Here's how the part is built. I have some questions about the finished solid (model axes, mm). Face numbers are marked on the shaded views. A direction names the side the tool comes from. Coordinates: 2 decimals unless noted, no trailing zeros. Write each loop counter-clockwise with the first axis right and the second up, starting at its lowest first coordinate (ties: lowest second). Pieces come first, ordered by that corner, then holes. Notation, with made-up numbers: (-18.75, 56) -> (5.25, 56) arc R11 cw to (5.25, 65) -> close; hole circle Ø8 at (70, -15.75). An arc over 180 degrees is marked (long way). Use CSV: the item, a comma, the result in double quotes. Start each with the question number.
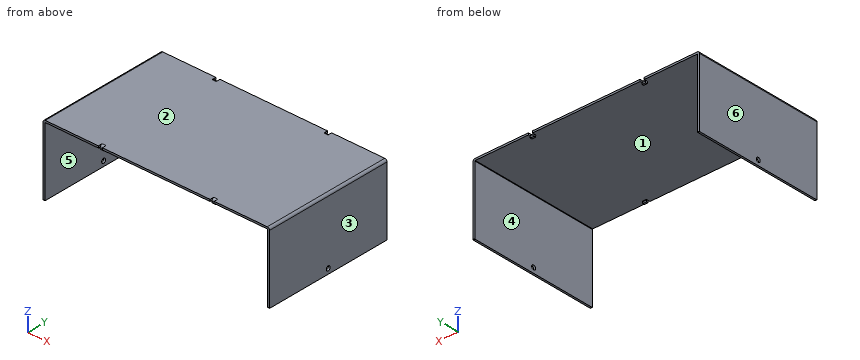
```python
from build123d import *

# Parameters (mm, degrees)
SKETCH1_W                      = 152.4
SKETCH1_H                      = 88.9
BASE_FLANGE1_DEPTH             = 1.29032
EDGE_FLANGE1_STRIP_W           = 5.85978
EDGE_FLANGE1_STRIP_H           = 1.29032
EDGE_FLANGE1_STRIP_CUT_DEPTH   = 88.9
EDGE_FLANGE1_STRIP_2_W         = 5.85978
EDGE_FLANGE1_STRIP_2_H         = 1.29032
EDGE_FLANGE1_STRIP_CUT_2_DEPTH = 88.9
EDGE_FLANGE1_DEPTH             = 88.9
EDGE_FLANGE1_BEND_DEPTH        = 88.9
M3X0_5_TAPPED_HOLE1_REACH      = 170.648
M3X0_5_TAPPED_HOLE1_BORE_R     = 1.5
BREAK_CORNER1_START            = -77.68082
BREAK_CORNER1_DEPTH            = 155.36164
CUT_THICKEN1_START             = 41.91
CUT_THICKEN1_OUTLINE_W         = 0.127
CUT_THICKEN1_OUTLINE_H         = 1.29032
CUT_THICKEN1_DEPTH             = 2.54
CUT_THICKEN2_START             = 41.91
CUT_THICKEN2_OUTLINE_W         = 0.127
CUT_THICKEN2_OUTLINE_H         = 1.29032
CUT_THICKEN2_DEPTH             = 2.54
MIRROR7_START                  = 41.91
MIRROR7_COPY_1_SKETCH_W        = 0.127
MIRROR7_COPY_1_SKETCH_H        = 1.29032
MIRROR7_COPY_1_DEPTH           = 2.54
MIRROR7_COPY_2_SKETCH_W        = 0.127
MIRROR7_COPY_2_SKETCH_H        = 1.29032
MIRROR7_COPY_2_DEPTH           = 2.54
MOVE_FACE1_BY                  = 1.27
MOVE_FACE1_2_BY                = 1.27
MOVE_FACE1_3_BY                = 1.27
MOVE_FACE1_4_BY                = 1.27
EDGE_FLANGE2_STRIP_W           = 5.66928
EDGE_FLANGE2_STRIP_H           = 1.29032
EDGE_FLANGE2_STRIP_CUT_DEPTH   = 2.54
EDGE_FLANGE2_STRIP_2_W         = 5.66928
EDGE_FLANGE2_STRIP_2_H         = 1.29032
EDGE_FLANGE2_STRIP_CUT_2_DEPTH = 2.54
EDGE_FLANGE2_STRIP_3_W         = 5.66928
EDGE_FLANGE2_STRIP_3_H         = 1.29032
EDGE_FLANGE2_STRIP_CUT_3_DEPTH = 2.54
EDGE_FLANGE2_STRIP_4_W         = 5.66928
EDGE_FLANGE2_STRIP_4_H         = 1.29032
EDGE_FLANGE2_STRIP_CUT_4_DEPTH = 2.54
EDGE_FLANGE2_DEPTH             = 2.54
EDGE_FLANGE2_BEND_DEPTH        = 2.54
EDGE_FLANGE2_BEND_2_DEPTH      = 2.54
EDGE_FLANGE2_BEND_3_DEPTH      = 2.54


# Read off the part's stored shape, not the designer's step: Break-Corner1, Cut-Thicken1, Cut-Thicken2
# Sheet-metal steps are written as plain solids
with BuildPart() as part:
    # Sketch1 → Base-Flange1 (new body)
    with BuildSketch(Plane.XY):
        Rectangle(SKETCH1_W, SKETCH1_H)
    extrude(amount=-BASE_FLANGE1_DEPTH)

    # Edge-Flange1 strip (across the edge) → Edge-Flange1 strip cut (cut)
    with BuildSketch(Plane(origin=(-76.3905, -44.45, -1.29032), x_dir=(1, 0, 0), z_dir=(0, 1, 0))):
        with Locations((-2.67589, -0.64516)):
            Rectangle(EDGE_FLANGE1_STRIP_W, EDGE_FLANGE1_STRIP_H)
    extrude(amount=EDGE_FLANGE1_STRIP_CUT_DEPTH, mode=Mode.SUBTRACT)

    # Edge-Flange1 strip 2 (across the edge) → Edge-Flange1 strip cut 2 (cut)
    with BuildSketch(Plane(origin=(76.3905, 44.45, -1.29032), x_dir=(-1, 0, 0), z_dir=(0, -1, 0))):
        with Locations((-2.67589, -0.64516)):
            Rectangle(EDGE_FLANGE1_STRIP_2_W, EDGE_FLANGE1_STRIP_2_H)
    extrude(amount=EDGE_FLANGE1_STRIP_CUT_2_DEPTH, mode=Mode.SUBTRACT)

    # Edge-Flange1 section (across the edge) → Edge-Flange1 (add)
    with BuildSketch(Plane(origin=(-76.3905, -44.45, -1.29032), x_dir=(1, 0, 0), z_dir=(0, 1, 0))):
        with BuildLine():
            Line((-1.29032, 0.254), (-1.29032, 46.96968))
            Line((-1.29032, 46.96968), (0, 46.96968))
            Line((0, 46.96968), (0, 0.254))
            ThreePointArc((0, 0.254), (0.074394878, 0.074394878), (0.254, 0))
            Line((0.254, 0), (0.254, -1.29032))
            ThreePointArc((0.254, -1.29032), (-0.837999144, -0.837999144), (-1.29032, 0.254))
        make_face()
    extrude(amount=EDGE_FLANGE1_DEPTH)

    # Edge-Flange1 section 2 (across the edge) → Edge-Flange1 bend (add)
    with BuildSketch(Plane(origin=(76.3905, 44.45, -1.29032), x_dir=(-1, 0, 0), z_dir=(0, -1, 0))):
        with BuildLine():
            Line((-1.29032, 0.254), (-1.29032, 46.96968))
            Line((-1.29032, 46.96968), (0, 46.96968))
            Line((0, 46.96968), (0, 0.254))
            ThreePointArc((0, 0.254), (0.074394878, 0.074394878), (0.254, 0))
            Line((0.254, 0), (0.254, -1.29032))
            ThreePointArc((0.254, -1.29032), (-0.837999144, -0.837999144), (-1.29032, 0.254))
        make_face()
    extrude(amount=EDGE_FLANGE1_BEND_DEPTH)

    # M3x0.5 Tapped Hole1 bore → M3x0.5 Tapped Hole1 (cut, up to next)
    with BuildSketch(Plane.ZY.offset(77.68082), mode=Mode.PRIVATE) as m3x0_5_tapped_hole1_sk1:
        with Locations((-44.7675, 0)):
            Circle(M3X0_5_TAPPED_HOLE1_BORE_R)
    m3x0_5_tapped_hole1_tool1 = extrude(m3x0_5_tapped_hole1_sk1.sketch, amount=-M3X0_5_TAPPED_HOLE1_REACH, mode=Mode.PRIVATE) & part.part
    m3x0_5_tapped_hole1 = m3x0_5_tapped_hole1_tool1.solids().sort_by_distance((-77.68082, 0, -44.7675))[0]
    add(m3x0_5_tapped_hole1, mode=Mode.SUBTRACT)

    # Mirror1: M3x0.5 Tapped Hole1 across plane
    add(m3x0_5_tapped_hole1.mirror(Plane(origin=(0, 0, 0), x_dir=(0, 0, 1), z_dir=(1, 0, 0))), mode=Mode.SUBTRACT)

    # Break-Corner1 outline → Break-Corner1 (cut)
    with BuildSketch(Plane.YZ.offset(BREAK_CORNER1_START)):
        with BuildLine():
            Line((44.45, -48.26), (44.45, -48.006))
            ThreePointArc((44.45, -48.006), (44.375605122, -48.185605122), (44.196, -48.26))
            Line((44.196, -48.26), (44.45, -48.26))
        make_face()
        with BuildLine():
            Line((-44.45, -48.26), (-44.196, -48.26))
            ThreePointArc((-44.196, -48.26), (-44.375605122, -48.185605122), (-44.45, -48.006))
            Line((-44.45, -48.006), (-44.45, -48.26))
        make_face()
    extrude(amount=BREAK_CORNER1_DEPTH, mode=Mode.SUBTRACT)

    # Cut-Thicken1 outline → Cut-Thicken1 (cut)
    with BuildSketch(Plane(origin=(0, 0, 0), x_dir=(1, 0, 0), z_dir=(0, 1, 0)).offset(CUT_THICKEN1_START)):
        with Locations((36.97732, 0.64516)):
            Rectangle(CUT_THICKEN1_OUTLINE_W, CUT_THICKEN1_OUTLINE_H)
    cut_thicken1 = extrude(amount=CUT_THICKEN1_DEPTH, mode=Mode.SUBTRACT)

    # Cut-Thicken2 outline → Cut-Thicken2 (cut)
    with BuildSketch(Plane(origin=(0, 0, 0), x_dir=(1, 0, 0), z_dir=(0, 1, 0)).offset(CUT_THICKEN2_START)):
        with Locations((39.64432, 0.64516)):
            Rectangle(CUT_THICKEN2_OUTLINE_W, CUT_THICKEN2_OUTLINE_H)
    cut_thicken2 = extrude(amount=CUT_THICKEN2_DEPTH, mode=Mode.SUBTRACT)

    # Mirror6: Cut-Thicken1, Cut-Thicken2 across plane
    add(cut_thicken1.mirror(Plane(origin=(0, 0, 0), x_dir=(0, 0, 1), z_dir=(1, 0, 0))), mode=Mode.SUBTRACT)
    add(cut_thicken2.mirror(Plane(origin=(0, 0, 0), x_dir=(0, 0, 1), z_dir=(1, 0, 0))), mode=Mode.SUBTRACT)

    # Mirror7: Cut-Thicken1, Cut-Thicken2 across plane
    add(cut_thicken1.mirror(Plane.ZX), mode=Mode.SUBTRACT)
    add(cut_thicken2.mirror(Plane.ZX), mode=Mode.SUBTRACT)

    # Mirror7 copy 1 sketch → Mirror7 copy 1 (cut)
    with BuildSketch(Plane(origin=(0, 0, 0), x_dir=(-1, 0, 0), z_dir=(0, -1, 0)).offset(MIRROR7_START)):
        with Locations((36.97732, 0.64516)):
            Rectangle(MIRROR7_COPY_1_SKETCH_W, MIRROR7_COPY_1_SKETCH_H)
    extrude(amount=MIRROR7_COPY_1_DEPTH, mode=Mode.SUBTRACT)

    # Mirror7 copy 2 sketch → Mirror7 copy 2 (cut)
    with BuildSketch(Plane(origin=(0, 0, 0), x_dir=(-1, 0, 0), z_dir=(0, -1, 0)).offset(MIRROR7_START)):
        with Locations((39.64432, 0.64516)):
            Rectangle(MIRROR7_COPY_2_SKETCH_W, MIRROR7_COPY_2_SKETCH_H)
    extrude(amount=MIRROR7_COPY_2_DEPTH, mode=Mode.SUBTRACT)

    # Move Face1: a face moved inward by 1.27
    extrude(part.faces().sort_by_distance((-38.31082, -44.45, -0.64516))[0], amount=MOVE_FACE1_BY, dir=(0, 1, 0), mode=Mode.SUBTRACT)

    # Move Face1 2: a face moved inward by 1.27
    extrude(part.faces().sort_by_distance((38.31082, -44.45, -0.64516))[0], amount=MOVE_FACE1_2_BY, dir=(0, 1, 0), mode=Mode.SUBTRACT)

    # Move Face1 3: a face moved inward by 1.27
    extrude(part.faces().sort_by_distance((-38.31082, 44.45, -0.64516))[0], amount=MOVE_FACE1_3_BY, dir=(0, -1, 0), mode=Mode.SUBTRACT)

    # Move Face1 4: a face moved inward by 1.27
    extrude(part.faces().sort_by_distance((38.31082, 44.45, -0.64516))[0], amount=MOVE_FACE1_4_BY, dir=(0, -1, 0), mode=Mode.SUBTRACT)

    # Edge-Flange2 strip (across the edge) → Edge-Flange2 strip cut (cut)
    with BuildSketch(Plane(origin=(37.04082, 43.18, -1.29032), x_dir=(0, -1, 0), z_dir=(1, 0, 0))):
        with Locations((-1.29032, -0.64516)):
            Rectangle(EDGE_FLANGE2_STRIP_W, EDGE_FLANGE2_STRIP_H)
    extrude(amount=EDGE_FLANGE2_STRIP_CUT_DEPTH, mode=Mode.SUBTRACT)

    # Edge-Flange2 strip 2 (across the edge) → Edge-Flange2 strip cut 2 (cut)
    with BuildSketch(Plane(origin=(-39.58082, 43.18, -1.29032), x_dir=(0, -1, 0), z_dir=(1, 0, 0))):
        with Locations((-1.29032, -0.64516)):
            Rectangle(EDGE_FLANGE2_STRIP_2_W, EDGE_FLANGE2_STRIP_2_H)
    extrude(amount=EDGE_FLANGE2_STRIP_CUT_2_DEPTH, mode=Mode.SUBTRACT)

    # Edge-Flange2 strip 3 (across the edge) → Edge-Flange2 strip cut 3 (cut)
    with BuildSketch(Plane(origin=(39.58082, -43.18, -1.29032), x_dir=(0, 1, 0), z_dir=(-1, 0, 0))):
        with Locations((-1.29032, -0.64516)):
            Rectangle(EDGE_FLANGE2_STRIP_3_W, EDGE_FLANGE2_STRIP_3_H)
    extrude(amount=EDGE_FLANGE2_STRIP_CUT_3_DEPTH, mode=Mode.SUBTRACT)

    # Edge-Flange2 strip 4 (across the edge) → Edge-Flange2 strip cut 4 (cut)
    with BuildSketch(Plane(origin=(-37.04082, -43.18, -1.29032), x_dir=(0, 1, 0), z_dir=(-1, 0, 0))):
        with Locations((-1.29032, -0.64516)):
            Rectangle(EDGE_FLANGE2_STRIP_4_W, EDGE_FLANGE2_STRIP_4_H)
    extrude(amount=EDGE_FLANGE2_STRIP_CUT_4_DEPTH, mode=Mode.SUBTRACT)

    # Edge-Flange2 section (across the edge) → Edge-Flange2 (add)
    with BuildSketch(Plane(origin=(37.04082, 43.18, -1.29032), x_dir=(0, -1, 0), z_dir=(1, 0, 0))):
        with BuildLine():
            Line((0, 0.254), (0, 1.27))
            Line((0, 1.27), (1.29032, 1.27))
            Line((1.29032, 1.27), (1.29032, 0.254))
            ThreePointArc((1.29032, 0.254), (1.364714878, 0.074394878), (1.54432, 0))
            Line((1.54432, 0), (1.54432, -1.29032))
            ThreePointArc((1.54432, -1.29032), (0.452320856, -0.837999144), (0, 0.254))
        make_face()
    extrude(amount=EDGE_FLANGE2_DEPTH)

    # Edge-Flange2 section 2 (across the edge) → Edge-Flange2 bend (add)
    with BuildSketch(Plane(origin=(-39.58082, 43.18, -1.29032), x_dir=(0, -1, 0), z_dir=(1, 0, 0))):
        with BuildLine():
            Line((0, 0.254), (0, 1.27))
            Line((0, 1.27), (1.29032, 1.27))
            Line((1.29032, 1.27), (1.29032, 0.254))
            ThreePointArc((1.29032, 0.254), (1.364714878, 0.074394878), (1.54432, 0))
            Line((1.54432, 0), (1.54432, -1.29032))
            ThreePointArc((1.54432, -1.29032), (0.452320856, -0.837999144), (0, 0.254))
        make_face()
    extrude(amount=EDGE_FLANGE2_BEND_DEPTH)

    # Edge-Flange2 section 3 (across the edge) → Edge-Flange2 bend 2 (add)
    with BuildSketch(Plane(origin=(39.58082, -43.18, -1.29032), x_dir=(0, 1, 0), z_dir=(-1, 0, 0))):
        with BuildLine():
            Line((0, 0.254), (0, 1.27))
            Line((0, 1.27), (1.29032, 1.27))
            Line((1.29032, 1.27), (1.29032, 0.254))
            ThreePointArc((1.29032, 0.254), (1.364714878, 0.074394878), (1.54432, 0))
            Line((1.54432, 0), (1.54432, -1.29032))
            ThreePointArc((1.54432, -1.29032), (0.452320856, -0.837999144), (0, 0.254))
        make_face()
    extrude(amount=EDGE_FLANGE2_BEND_2_DEPTH)

    # Edge-Flange2 section 4 (across the edge) → Edge-Flange2 bend 3 (add)
    with BuildSketch(Plane(origin=(-37.04082, -43.18, -1.29032), x_dir=(0, 1, 0), z_dir=(-1, 0, 0))):
        with BuildLine():
            Line((0, 0.254), (0, 1.27))
            Line((0, 1.27), (1.29032, 1.27))
            Line((1.29032, 1.27), (1.29032, 0.254))
            ThreePointArc((1.29032, 0.254), (1.364714878, 0.074394878), (1.54432, 0))
            Line((1.54432, 0), (1.54432, -1.29032))
            ThreePointArc((1.54432, -1.29032), (0.452320856, -0.837999144), (0, 0.254))
        make_face()
    extrude(amount=EDGE_FLANGE2_BEND_3_DEPTH)


solid = part.part
```
Item 1: Thinking about a two-plate mould opening in X: for the marked faces 1, 2, 3 and 4, which applies, +X half, -X half, draft (parallel to the pull), parting line (faces both ways), or undercut?
Item 2: I'm going to push flat-ended pins straight in: pin 1 (8 mm diameter, centred on x = -21.5, y = -28.5, fed in from -Z); pin 2 (0.6 mm diameter, centred on x = 39, y = -43, fed in from -Z); pin 3 (0.8 mm diameter, centred on x = 37.5, z = -2, fed in from -Y). Where does each tip first touch, or does it pass through?
Item 3: I want a section at A-A on z = -37.5. Please give me the cut outline in (x, y), then the cut area to 3 significant figures.
Item 4: I want a section at D-D on x = 57.5. Please give me the cut outline in (y, z).
Item 5: I want a section at C-C on y = 14.5. Please give me the cut outline in (x, z).
Item 6: I want a section at B-B on y = 0. Please give me the cut outline in (x, z).
Item 7: Which directions (+Z, -Z, +X, -X, +Y, -Y) give clear straight access to the entire face, cutting with the end or side of a thin tool? Please do the marked faces 5 and 6.
Item 8: If I drill on line 1 along X through (y, z) = (6, -9.5); line 2 along Z through (x, y) = (-33.5, -14), over which ranges is the centre line in solid material (lowest first)?
Geometry says:
1,face 1,"undercut"
1,face 2,"draft"
1,face 3,"+X half"
1,face 4,"undercut"
2,pin 1,"z = -1.29"
2,pin 2,"z = -2.56"
2,pin 3,"y = -43.18"
3,outline,"(-77.68, -44.45) -> (-76.39, -44.45) -> (-76.39, 44.45) -> (-77.68, 44.45) -> close; (76.39, -44.45) -> (77.68, -44.45) -> (77.68, 44.45) -> (76.39, 44.45) -> close"
3,area,"229 mm2"
4,outline,"(-44.45, -1.29) -> (44.45, -1.29) -> (44.45, 0) -> (-44.45, 0) -> close"
5,outline,"(-77.68, -48.26) -> (-76.39, -48.26) -> (-76.39, -1.54) arc R0.25 cw to (-76.14, -1.29) -> (76.14, -1.29) arc R0.25 cw to (76.39, -1.54) -> (76.39, -48.26) -> (77.68, -48.26) -> (77.68, -1.54) arc R1.54 ccw to (76.14, 0) -> (-76.14, 0) arc R1.54 ccw to (-77.68, -1.54) -> close"
6,outline,"(-77.68, -48.26) -> (-76.39, -48.26) -> (-76.39, -46.27) -> (-77.68, -46.27) -> close; (-77.68, -43.27) -> (-76.39, -43.27) -> (-76.39, -1.54) arc R0.25 cw to (-76.14, -1.29) -> (76.14, -1.29) arc R0.25 cw to (76.39, -1.54) -> (76.39, -43.27) -> (77.68, -43.27) -> (77.68, -1.54) arc R1.54 ccw to (76.14, 0) -> (-76.14, 0) arc R1.54 ccw to (-77.68, -1.54) -> close; (76.39, -48.26) -> (77.68, -48.26) -> (77.68, -46.27) -> (76.39, -46.27) -> close"
7,face 5,"-Z, +Y, -Y"
7,face 6,"+Z, -Z, -X, +Y, -Y"
8,line 1,"-77.68 to -76.39, 76.39 to 77.68"
8,line 2,"-1.29 to 0"
